Geometry check sheet. Reference: the model listing, model coordinates, mm. Face numbers are marked on the shaded views. A direction names the side the tool comes from. Coordinates: 2 decimals unless noted, no trailing zeros. Order: outer loops, then holes, each group sorted by start corner. A loop starts at its lowest first (then second) coordinate and runs counter-clockwise, first axis right, second up. Notation, with made-up numbers: (42.25, 68) -> (65.25, 68) arc R8 ccw to (65.25, 76) -> close; hole circle Ø11 at (-26.75, -32). An arc over 180 degrees is marked (long way). Answer in a Markdown table with one row per item. Add a question column.
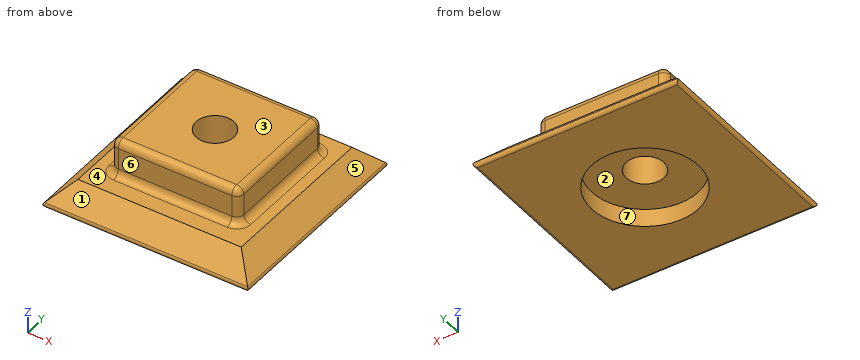
```python
from build123d import *

# Parameters (mm, degrees)
F0_W      = 38.1
F0_H      = 38.1
F1_DEPTH  = 4.445
F4_DEPTH  = 38.101
F5_DEPTH  = 38.101
F6_R      = 0.508
F7_W      = 22.86
F7_H      = 21.9536569705
F8_DEPTH  = 6.35
F9_R      = 3.3734375
F10_DEPTH = 10.7965917968
F11_R     = 9.525
F12_DEPTH = 3.175
F13_R     = 1.27


with BuildPart() as f1:
    # F0 (on Top) → F1 (new body)
    with BuildSketch(Plane.XY):
        Rectangle(F0_W, F0_H)
    extrude(amount=F1_DEPTH)

    # F2 (on face) → F4 (cut, through all)
    with BuildSketch(Plane.XZ.offset(19.05)):
        Polygon((-19.05, 4.445), (-19.05, 0), (-14.605, 4.445), align=None)
        Polygon((14.605, 4.445), (19.05, 0), (19.05, 4.445), align=None)
    extrude(amount=-F4_DEPTH, mode=Mode.SUBTRACT)

    # F3 (on face) → F5 (cut, through all)
    with BuildSketch(Plane(origin=(-19.05, 0, 0), x_dir=(0, -1, 0), z_dir=(-1, 0, 0))):
        Polygon((-19.05, 4.445), (-19.05, 0), (-14.605, 4.445), align=None)
        Polygon((14.605, 4.445), (19.05, 0), (19.05, 4.445), align=None)
    extrude(amount=-F5_DEPTH, mode=Mode.SUBTRACT)

    # F6
    f6_edges = [f1.edges().sort_by_distance(p)[0] for p in [
        (19.05, 0, 0),
        (0, -19.05, 0),
        (-19.05, 0, 0),
        (0, 19.05, 0),
    ]]
    fillet(f6_edges, radius=F6_R)

    # F7 (on face) → F8 (join)
    with BuildSketch(Plane.XY.offset(4.445)):
        with Locations((0, 0.4531715147)):
            Rectangle(F7_W, F7_H)
    extrude(amount=F8_DEPTH)

    # F9 (on face) → F10 (cut, through all)
    with BuildSketch(Plane.XY.offset(10.795)):
        Circle(F9_R)
    extrude(amount=-F10_DEPTH, mode=Mode.SUBTRACT)

    # F11 (on face) → F12 (cut)
    with BuildSketch(Plane(origin=(0, 0, 0), x_dir=(1, 0, 0), z_dir=(0, 0, -1))):
        Circle(F11_R)
    extrude(amount=-F12_DEPTH, mode=Mode.SUBTRACT)

    # F13
    f13_edges = [f1.edges().sort_by_distance(p)[0] for p in [
        (-11.43, 0.453172, 4.445),
        (0, -10.523657, 4.445),
        (-11.43, -10.523657, 7.62),
        (-11.43, 11.43, 7.62),
        (11.43, 11.43, 7.62),
        (11.43, -10.523657, 7.62),
        (0, 11.43, 10.795),
        (11.43, 0.453172, 10.795),
        (0, -10.523657, 10.795),
        (-18.18279, 0, 0.86721),
        (-11.43, 0.453172, 10.795),
        (11.43, 0.453172, 4.445),
        (0, 11.43, 4.445),
    ]]
    fillet(f13_edges, radius=F13_R)


solid = f1.part
```
(1) Mould release check, pull along Y, two halves, no side actions. Record for the marked faces 1, 2 and 3: +Y half, -Y half, draft (parallel to the pull), parting line (faces both ways), or undercut.
(2) Cross-section at D-D (z = 1.75). Enter the section's corners in (x, y) (3 decimals).
(3) Access from +Z, -Z, +X, -X, +Y, -Y to the whole of each face (thin tool, end or side, straight path). Record for the marked faces 4, 5, 6 and 7.
(4) Scan lines: line 1 along Y through (x, z) = (0, 9); line 2 along X through (y, z) = (0, 0.8) (3 decimals); line 3 along Z through (x, y) = (-7, 3.5) (3 decimals). Record each from-to range of solid material in increasing order.
(5) Cross-section at B-B (y = 0). Enter the section's corners in (x, z) (3 decimals), plus the area to 3 significant figures.
(6) Cross-section at C-C (x = 0). Enter the section's corners in (y, z) (3 decimals), plus the area to 3 significant figures.
(7) Cross-section at A-A (z = 8.25). Enter the section's corners in (x, y).
(8) Go/stop test with flat-tipped pins: P1, Ø4, axis at x = -1.5, z = 7.5, coming from the +Y side; P2, Ø1, axis at y = 6.5, z = 7, coming from the -X side; P3, Ø3, axis at y = 11.5, z = 4.5, coming from the -X side. Record where each tip stops, or that it passes through.
Checks:
| question | item | result |
|---|---|---|
| 1 | face 1 | -Y half |
| 1 | face 2 | undercut |
| 1 | face 3 | draft |
| 2 | outline | (-17.3, -17.3) -> (17.3, -17.3) -> (17.3, 17.3) -> (-17.3, 17.3) -> close; hole circle Ø19.05 at (0, 0) |
| 3 | face 4 | +Z |
| 3 | face 5 | +Z, +X, +Y, -Y |
| 3 | face 6 | +Z, +X, -X, -Y |
| 3 | face 7 | -Z |
| 4 | line 1 | -10.52 to -3.37, 3.37 to 11.43 |
| 4 | line 2 | -18.239 to -9.525, 9.525 to 18.239 |
| 4 | line 3 | 3.175 to 10.795 |
| 5 | outline | (-18.183, 0.867) arc R0.508 ccw to (-17.824, 0) -> (-9.525, 0) -> (-9.525, 3.175) -> (-3.373, 3.175) -> (-3.373, 10.795) -> (-10.16, 10.795) arc R1.27 ccw to (-11.43, 9.525) -> (-11.43, 5.715) arc R1.27 cw to (-12.7, 4.445) -> (-14.605, 4.445) -> close; (3.373, 3.175) -> (9.525, 3.175) -> (9.525, 0) -> (17.824, 0) arc R0.508 ccw to (18.183, 0.867) -> (14.605, 4.445) -> (12.7, 4.445) arc R1.27 cw to (11.43, 5.715) -> (11.43, 9.525) arc R1.27 ccw to (10.16, 10.795) -> (3.373, 10.795) -> close |
| 5 | area | 182 mm² |
| 6 | outline | (-18.183, 0.867) arc R0.508 ccw to (-17.824, 0) -> (-9.525, 0) -> (-9.525, 3.175) -> (-3.373, 3.175) -> (-3.373, 10.795) -> (-9.254, 10.795) arc R1.27 ccw to (-10.524, 9.525) -> (-10.524, 5.715) arc R1.27 cw to (-11.794, 4.445) -> (-14.605, 4.445) -> close; (3.373, 3.175) -> (9.525, 3.175) -> (9.525, 0) -> (17.824, 0) arc R0.508 ccw to (18.183, 0.867) -> (14.605, 4.445) -> (12.7, 4.445) arc R1.27 cw to (11.43, 5.715) -> (11.43, 9.525) arc R1.27 ccw to (10.16, 10.795) -> (3.373, 10.795) -> close |
| 6 | area | 176 mm² |
| 7 | outline | (-11.43, -9.25) arc R1.27 ccw to (-10.16, -10.52) -> (10.16, -10.52) arc R1.27 ccw to (11.43, -9.25) -> (11.43, 10.16) arc R1.27 ccw to (10.16, 11.43) -> (-10.16, 11.43) arc R1.27 ccw to (-11.43, 10.16) -> close; hole circle Ø6.75 at (0, 0) |
| 8 | P1 | y = 11.45 |
| 8 | P2 | x = -11.43 |
| 8 | P3 | x = -16.05 |
